Verification items for this drawing (mm, ordinates from the low corner). A direction names the side the tool comes from. Coordinates: 2 decimals unless noted, no trailing zeros. Order: outer loops, then holes, each group sorted by start corner. A loop starts at its lowest first (then second) coordinate and runs counter-clockwise, first axis right, second up. Notation, with made-up numbers: (-22.75, 30) - (-13.75, 30) arc R22 ccw to (-13.75, 54) - close; hole circle Ø1 at (78.25, -38.5). An arc over 180 degrees is marked (long way). One line per question, with ' | ' between items. Start each with the question number.
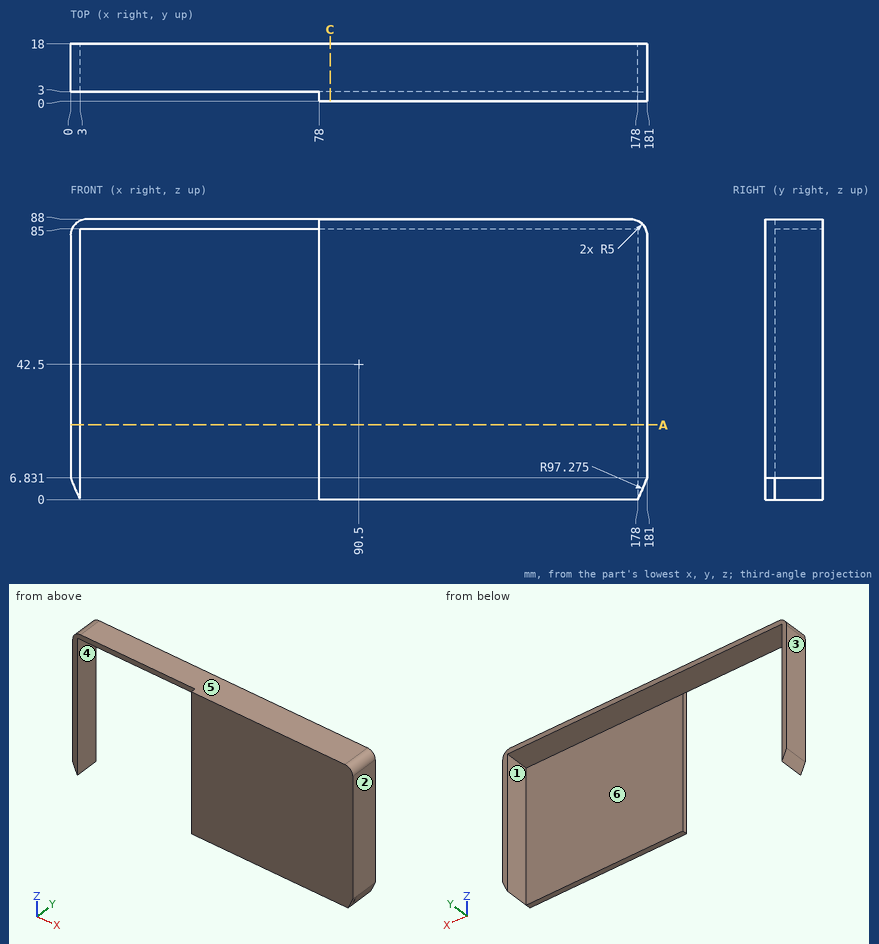
Item 1: Set-up check for the marked faces 4, 5 and 6: record each of +Z, -Z, +X, -X, +Y, -Y from which the full face is reachable in a straight line by a thin tool's end or side.
Item 2: Section check C-C (x = 81.5). Record the cut outline in (y, z), then the cut area to 3 significant figures.
Item 3: Section check A-A (z = 23.5). Record the cut outline in (x, y).
Item 4: Mould release check, pull along X, two halves, no side actions. Record for the marked faces 1, 2 and 3: +X half, -X half, draft (parallel to the pull), parting line (faces both ways), or undercut.
Item 5: Thickness scan on probe 1 along X at (y, z) = (4.75, 20.5); probe 2 along Z at (x, y) = (102, 12.5); probe 3 along Y at (x, z) = (88, 34). Record the ranges inside material, lowest first. Write a range as from..to.
Item 6: Gauge pin test, flat ends, axial feed: pin 1 (3 mm diameter, centred on x = 117.5, z = 63.5, fed in from +Y); pin 2 (1 mm diameter, centred on x = 98.5, y = 14.5, fed in from -Z). Record the tip position at first contact, or that the pin passes through.
Completed:
1) face 4: -Z, +Y, -Y | face 5: +Z, +X, -X, +Y, -Y | face 6: -Z, +Y
2) outline: (0, 0) - (3, 0) - (3, 85) - (18, 85) - (18, 88) - (0, 88) - close | area: 309 mm^2
3) outline: (0, 3) - (3, 3) - (3, 18) - (0, 18) - close; (78, 0) - (181, 0) - (181, 18) - (178, 18) - (178, 3) - (78, 3) - close
4) face 1: undercut | face 2: +X half | face 3: -X half
5) probe 1: x = 0..3, 178..181 | probe 2: z = 85..88 | probe 3: y = 0..3
6) pin 1: stops at y = 3 | pin 2: stops at z = 85
